```python
from build123d import *

# Parameters (mm, degrees)
SKETCH1_R            = 16.4
BOSS_EXTRUDE1_DEPTH  = 23
SKETCH2_R            = 1.25
BOSS_EXTRUDE2_DEPTH  = 0.5
SKETCH4_R            = 18.5
BOSS_EXTRUDE4_DEPTH  = 22.8
CUT_EXTRUDE1_DEPTH   = 1
SKETCH6_R            = 6.006706661
BOSS_EXTRUDE5_DEPTH  = 6
SKETCH7_R            = 3
BOSS_EXTRUDE6_DEPTH  = 15
CUT_EXTRUDE2_START   = -12
CUT_EXTRUDE2_DEPTH   = 12
BOSS_EXTRUDE7_DEPTH  = 0.8
REVOLVE4_ANGLE       = 180
SKETCH13_R           = 1
BOSS_EXTRUDE9_DEPTH  = 2.5
SKETCH14_R           = 6.75
BOSS_EXTRUDE10_DEPTH = 5.5
SKETCH15_W           = 7.5
SKETCH15_H           = 16
BOSS_EXTRUDE11_DEPTH = 5.5


with BuildPart() as part:
    # Sketch1 → Boss-Extrude1 (new body)
    with BuildSketch(Plane(origin=(0, 0, 0), x_dir=(-1, 0, 0), z_dir=(0, 1, 0))):
        with Locations(Location((0, 0, 0), (0, 0, 90))):
            Circle(SKETCH1_R)
    extrude(amount=BOSS_EXTRUDE1_DEPTH)

    # Sketch2 → Boss-Extrude2 (add)
    with BuildSketch(Plane(origin=(0, 23, 0), x_dir=(-1, 0, 0), z_dir=(0, 1, 0))):
        with Locations(Location((0, 12.5, 0), (0, 0, 90))):
            Circle(SKETCH2_R)
        with Locations(Location((0, -12.5, 0), (0, 0, 90))):
            Circle(SKETCH2_R)
    extrude(amount=BOSS_EXTRUDE2_DEPTH)

    # Sketch4 → Boss-Extrude4 (add)
    with BuildSketch(Plane.XZ):
        with Locations(Location((0, 0, 0), (0, 0, 270))):
            Circle(SKETCH4_R)
    extrude(amount=BOSS_EXTRUDE4_DEPTH)

    # Sketch5 → Cut-Extrude1 (cut)
    with BuildSketch(Plane.XZ.offset(22.8)):
        with BuildLine():
            ThreePointArc((-8.811209519, 8.866373938), (0, -12.5), (8.811209519, 8.866373938))
            ThreePointArc((8.811209519, 8.866373938), (0, -2.006706661), (-8.811209519, 8.866373938))
        make_face()
    extrude(amount=-CUT_EXTRUDE1_DEPTH, mode=Mode.SUBTRACT)

    # Sketch6 → Boss-Extrude5 (add)
    with BuildSketch(Plane.XZ.offset(22.8)):
        with Locations(Location((0, 7, 0), (0, 0, 270))):
            Circle(SKETCH6_R)
    extrude(amount=BOSS_EXTRUDE5_DEPTH)

    # Sketch7 → Boss-Extrude6 (add)
    with BuildSketch(Plane.XZ.offset(28.8)):
        with Locations(Location((0, 7, 0), (0, 0, 270))):
            Circle(SKETCH7_R)
    extrude(amount=BOSS_EXTRUDE6_DEPTH)

    # Sketch8 → Cut-Extrude2 (cut)
    with BuildSketch(Plane.XZ.offset(43.8).offset(CUT_EXTRUDE2_START)):
        with BuildLine():
            Line((-1.8, 9.4), (1.8, 9.4))
            ThreePointArc((1.8, 9.4), (0, 10), (-1.8, 9.4))
        make_face()
    extrude(amount=CUT_EXTRUDE2_DEPTH, mode=Mode.SUBTRACT)

    # Sketch9 → Boss-Extrude7 (add)
    with BuildSketch(Plane(origin=(0, 23.5, 0), x_dir=(-1, 0, 0), z_dir=(0, 1, 0))):
        with BuildLine():
            Line((-12.680693987, 10.4), (-16.4, 10.4))
            Line((-16.4, 10.4), (-16.4, -10.4))
            Line((-16.4, -10.4), (-12.680693987, -10.4))
            ThreePointArc((-12.680693987, -10.4), (16.4, 0), (-12.680693987, 10.4))
        make_face()
    extrude(amount=BOSS_EXTRUDE7_DEPTH)

    # Sketch10 → Revolve4 (revolve)
    with BuildSketch(Plane(origin=(0, 24.3, 0), x_dir=(-1, 0, 0), z_dir=(0, 1, 0))):
        with BuildLine():
            Line((0, 13.75), (0, 11.25))
            ThreePointArc((0, 11.25), (1.25, 12.5), (0, 13.75))
        make_face()
        with BuildLine():
            Line((0, -11.25), (0, -13.75))
            ThreePointArc((0, -13.75), (1.25, -12.5), (0, -11.25))
        make_face()
    revolve(axis=Axis((0, 24.3, 12.5), (0, 0, -1)), revolution_arc=REVOLVE4_ANGLE)

    # Sketch13 → Boss-Extrude9 (add)
    with BuildSketch(Plane(origin=(0, 24.3, 0), x_dir=(-1, 0, 0), z_dir=(0, 1, 0))):
        with Locations(Location((0, 0, 0), (0, 0, 270))):
            Circle(SKETCH13_R)
    extrude(amount=BOSS_EXTRUDE9_DEPTH)

    # Sketch14 → Boss-Extrude10 (add)
    with BuildSketch(Plane(origin=(0, 26.8, 0), x_dir=(-1, 0, 0), z_dir=(0, 1, 0))):
        with Locations(Location((0, 0, 0), (0, 0, 90))):
            Circle(SKETCH14_R)
    extrude(amount=BOSS_EXTRUDE10_DEPTH)

    # Sketch15 → Boss-Extrude11 (add)
    with BuildSketch(Plane(origin=(0, 24.3, 0), x_dir=(-1, 0, 0), z_dir=(0, 1, 0))):
        with Locations((-12.15, 0)):
            Rectangle(SKETCH15_W, SKETCH15_H)
    extrude(amount=BOSS_EXTRUDE11_DEPTH)


solid = part.part
```
CAD build for the part. Positions are in the model's coordinates, mm. A direction names the side the tool comes from. Coordinates: 2 decimals unless noted, no trailing zeros. Order: outer loops, then holes, each group sorted by start corner. A loop starts at its lowest first (then second) coordinate and runs counter-clockwise, first axis right, second up. Notation, with made-up numbers: M 10,41 L 41,41 A20 ccw 41,71 Z; hole C 36,83.25 d10. An arc over 180 degrees is marked long. Answer as CSV lines item,"result".
1) Cut at D-D (z = -4.5). List the corners of the cut face in (x, y).
Verdict:
outline,"M -17.94,-22.8 L -11.66,-22.8 L -11.66,-21.8 L 11.66,-21.8 L 11.66,-22.8 L 17.94,-22.8 L 17.94,0 L 15.77,0 L 15.77,23 L -15.77,23 L -15.77,0 L -17.94,0 Z; M -15.77,23.5 L 16.4,23.5 L 16.4,24.3 L 15.9,24.3 L 15.9,29.8 L 8.4,29.8 L 8.4,24.3 L -15.77,24.3 Z; M -5.03,26.8 L 5.03,26.8 L 5.03,32.3 L -5.03,32.3 Z"
2) Cut at B-B (z = 3). Give the number of separate pieces and of enclosed holes in the cut face, then the cut area to 3 significant figures.
Verdict:
separate pieces,"3"
enclosed holes,"0"
area,"1,750 mm2"
3) Drill centre lines: L1, parallel to Y at x = -2, z = 3; L2, parallel to Y at x = -4.5, z = -8.5; L3, parallel to X at y = -22, z = 0. Where is each one in solid material? Low to high. Write a range as from..to.
Verdict:
L1,"-28.8..23, 23.5..24.3, 26.8..32.3"
L2,"-21.8..23, 23.5..24.3"
L3,"-18.5..-12.5, -5.67..5.67, 12.5..18.5"
4) Flat gauge pins, fed straight in: P1, Ø10, axis at x = -14, y = -30.5, coming from the -Z side; P2, Ø5, axis at x = -3, z = -3, coming from the -Y side; P3, Ø6, axis at x = 11.5, z = -3.5, coming from the +Y side; P4, Ø1, axis at x = -8.5, z = -8.5, coming from the +Y side. Where does each tip first touch, or does it go through?
Verdict:
P1,"through"
P2,"y = -22.8"
P3,"y = 29.8"
P4,"y = 24.3"
5) Mould opens along Z. For faces 1 (the cylindrical face through (0.224, -22.307, -2.004)), 2 (the flat face through (12, 27, -8)), 3 (the flat face through (-15, 0, 7)) say: released by +Z, released by -Z, zero draft, split by the parting line, or undercut.
Verdict:
face 1,"undercut"
face 2,"released by -Z"
face 3,"zero draft"
6) Cut at A-A (x = -15). List the corners of the cut face in (y, z), then the cut area to 3 significant figures.
Verdict:
outline,"M -22.8,-10.83 L 0,-10.83 L 0,-6.63 L 23,-6.63 L 23,6.63 L 0,6.63 L 0,10.83 L -22.8,10.83 Z; M 23.5,-6.63 L 24.3,-6.63 L 24.3,6.63 L 23.5,6.63 Z"
area,"809 mm2"
7) 3-axis set-ups, long thin cutter, end or side, ignore diameter. For faces 4 (the flat face through (-1, -28.8, 10)), 5 (the cylindrical face through (-16.39, 23.89, -0.56)), 6 (the flat face through (0, -43.8, 7)), 7 (the cylindrical face through (16.26, 11.34, -2.13)), 8 (the flat face through (12, 29.8, 0)): which of +Z, -Z, +X, -X, +Y, -Y reach the whole face in a straight line?
Verdict:
face 4,"-Y"
face 5,"+Y"
face 6,"+Z, -Z, +X, -X, -Y"
face 7,"none"
face 8,"+Z, -Z, +X, +Y"
8) Cut at C-C (y = 12). List the corners of the cut face in (x, z).
Verdict:
outline,"C 0,0 d32.8"
